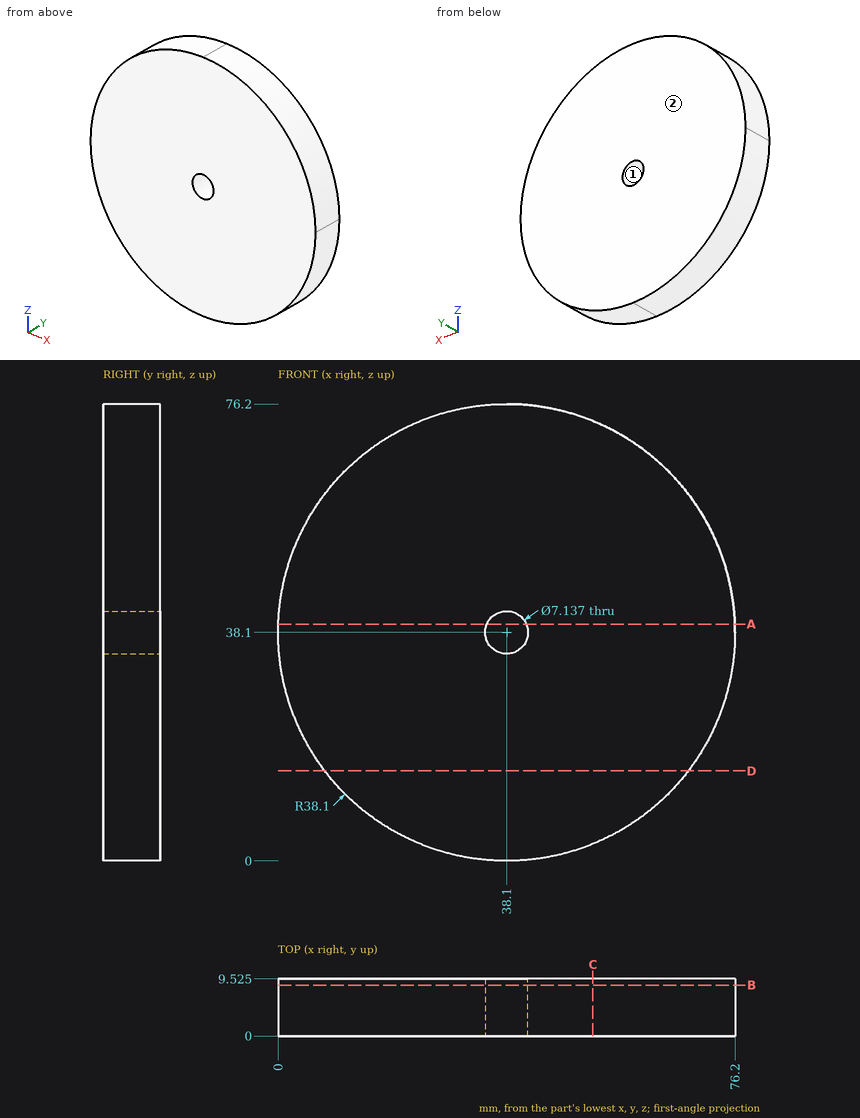
The drawing under review shows one solid part. Ordinate dimensions are in mm from its lowest x, y, z. Coordinates: 2 decimals unless noted, no trailing zeros. Write each loop counter-clockwise with the first axis right and the second up, starting at its lowest first coordinate (ties: lowest second). Pieces come first, ordered by that corner, then holes. Notation, with made-up numbers: M -40,61 L -25,61 A10 ccw -25,67 Z; hole C 1.5,9.5 d9. An arc over 180 degrees is marked long. Put each result on its own line as item: value.
1) Clearance check with flat-ended pins moving along their axes: pin 1 Ø5 at (x, y) = (13, 5) entering from +Z; pin 2 Ø2 at (x, y) = (51, 6.5) entering from +Z. State where each tip first meets the part, or that it passes through.
Computed:
pin 1: stops at z = 68.77
pin 2: stops at z = 74.29
2) Add section A-A on z = 39.5. Give the boundary of the cut face in (x, y) (1 decimal), then the cut area to 3 significant figures.
Computed:
outline: M 0,0 L 34.8,0 L 34.8,9.5 L 0,9.5 Z; M 41.4,0 L 76.2,0 L 76.2,9.5 L 41.4,9.5 Z
area: 663 mm2
3) Wall thickness on probe 1 along Z at (x, y) = (38.1, 2.5); probe 2 along X at (y, z) = (8.25, 36.5) (1 decimal); probe 3 along X at (y, z) = (1.25, 40.5) (1 decimal): over which ranges is each line inside the solid? List them lowest first. Write a range as [from, to].
Computed:
probe 1: z = [0, 34.53], [41.67, 76.2]
probe 2: x = [0, 34.9], [41.3, 76.2]
probe 3: x = [0.1, 35.5], [40.7, 76.1]
4) Add section B-B on y = 8.5. Give the boundary of the cut face in (x, z), then the cut area to 3 significant figures.
Computed:
outline: C 38.1,38.1 d76.2; hole C 38.1,38.1 d7.14
area: 4,520 mm2
5) Draft analysis for pull direction X (two halves, no side actions). For the marked faces 1 and 2, state which applies: released by +X, released by -X, zero draft, split by the parting line, or undercut.
Computed:
face 1: undercut
face 2: zero draft
6) Add section D-D on z = 15. Give the boundary of the cut face in (x, y) (1 decimal).
Computed:
outline: M 7.8,0 L 68.4,0 L 68.4,9.5 L 7.8,9.5 Z
7) Add section C-C on x = 52.5. Give the boundary of the cut face in (y, z) (1 decimal).
Computed:
outline: M 0,2.8 L 9.5,2.8 L 9.5,73.4 L 0,73.4 Z
